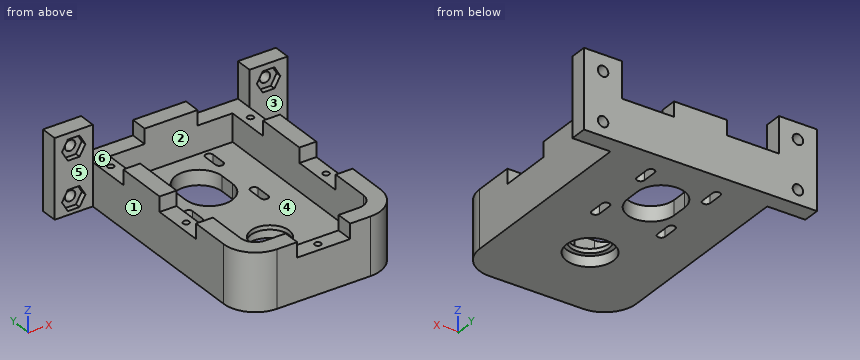
```python
from build123d import *

# Parameters (mm, degrees)
CROQUIS2_R                = 9
SALIENTE_EXTRUIR1_DEPTH   = 7
CROQUIS2_5_W              = 18
CROQUIS2_5_H              = 8
SALIENTE_EXTRUIR2_DEPTH   = 37
SALIENTE_EXTRUIR2_2_DEPTH = 37
CROQUIS2_7_W              = 25
CROQUIS2_7_H              = 8
CROQUIS2_7_W_2            = 8
CROQUIS2_7_H_2            = 25
CROQUIS2_7_H_3            = 19
CROQUIS2_7_W_3            = 9.5
SALIENTE_EXTRUIR3_DEPTH   = 27
CROQUIS2_8_W              = 8
CROQUIS2_8_H              = 25
CROQUIS2_8_W_2            = 25
CROQUIS2_8_H_2            = 8
SALIENTE_EXTRUIR4_DEPTH   = 20
CROQUIS3_R                = 11.1
CORTAR_EXTRUIR1_DEPTH     = 5
CROQUIS9_R                = 2.475
CORTAR_EXTRUIR2_DEPTH     = 2.5
CROQUIS10_R               = 2.475
CORTAR_EXTRUIR3_DEPTH     = 8
CROQUIS11_R               = 1.475
CORTAR_EXTRUIR4_DEPTH     = 7


with BuildPart() as part:
    # Croquis2 → Saliente-Extruir1 (new body)
    with BuildSketch(Plane.XY):
        with BuildLine():
            Line((-5.786620614, -56.183989891), (3.713379386, -56.183989891))
            ThreePointArc((3.713379386, -56.183989891), (8.663126854, -54.133737359), (10.713379386, -49.183989891))
            Line((10.713379386, -49.183989891), (10.713379386, -30.183989891))
            Line((10.713379386, -30.183989891), (10.713379386, -5.183989891))
            Line((10.713379386, -5.183989891), (10.713379386, 19.816010109))
            Line((10.713379386, 19.816010109), (10.713379386, 40.816010109))
            Line((10.713379386, 40.816010109), (-5.786620614, 40.816010109))
            Line((-5.786620614, 40.816010109), (-30.786620614, 40.816010109))
            Line((-30.786620614, 40.816010109), (-47.286620614, 40.816010109))
            Line((-47.286620614, 40.816010109), (-47.286620614, 19.816010109))
            Line((-47.286620614, 19.816010109), (-47.286620614, -5.183989891))
            Line((-47.286620614, -5.183989891), (-47.286620614, -30.183989891))
            Line((-47.286620614, -30.183989891), (-47.286620614, -49.183989891))
            ThreePointArc((-47.286620614, -49.183989891), (-45.236368082, -54.133737359), (-40.286620614, -56.183989891))
            Line((-40.286620614, -56.183989891), (-30.786620614, -56.183989891))
            Line((-30.786620614, -56.183989891), (-5.786620614, -56.183989891))
        make_face()
        with Locations((-18.286620614, -27.183989891)):
            Circle(CROQUIS2_R, mode=Mode.SUBTRACT)
        with BuildLine():
            ThreePointArc((-31.986620614, 6.205288522), (-33.786620614, 8.005288522), (-35.586620614, 6.205288522))
            Line((-35.586620614, 6.205288522), (-35.586620614, -0.794711478))
            ThreePointArc((-35.586620614, -0.794711478), (-33.786620614, -2.594711478), (-31.986620614, -0.794711478))
            Line((-31.986620614, -0.794711478), (-31.986620614, 6.205288522))
        make_face(mode=Mode.SUBTRACT)
        with BuildLine():
            ThreePointArc((-4.586620614, 30.205288522), (-2.786620614, 28.405288522), (-0.986620614, 30.205288522))
            Line((-0.986620614, 30.205288522), (-0.986620614, 37.205288522))
            ThreePointArc((-0.986620614, 37.205288522), (-2.786620614, 39.005288522), (-4.586620614, 37.205288522))
            Line((-4.586620614, 37.205288522), (-4.586620614, 30.205288522))
        make_face(mode=Mode.SUBTRACT)
        with BuildLine():
            ThreePointArc((-29.286620614, 14.705288522), (-18.286620614, 3.705288522), (-7.286620614, 14.705288522))
            Line((-7.286620614, 14.705288522), (-7.286620614, 21.705288522))
            ThreePointArc((-7.286620614, 21.705288522), (-18.286620614, 32.705288522), (-29.286620614, 21.705288522))
            Line((-29.286620614, 21.705288522), (-29.286620614, 14.705288522))
        make_face(mode=Mode.SUBTRACT)
        with BuildLine():
            Line((-0.986620614, 6.205288522), (-0.986620614, -0.794711478))
            ThreePointArc((-0.986620614, -0.794711478), (-2.786620614, -2.594711478), (-4.586620614, -0.794711478))
            Line((-4.586620614, -0.794711478), (-4.586620614, 6.205288522))
            ThreePointArc((-4.586620614, 6.205288522), (-2.786620614, 8.005288522), (-0.986620614, 6.205288522))
        make_face(mode=Mode.SUBTRACT)
        with BuildLine():
            Line((-35.586620614, 30.205288522), (-35.586620614, 37.205288522))
            ThreePointArc((-35.586620614, 37.205288522), (-33.786620614, 39.005288522), (-31.986620614, 37.205288522))
            Line((-31.986620614, 37.205288522), (-31.986620614, 30.205288522))
            ThreePointArc((-31.986620614, 30.205288522), (-33.786620614, 28.405288522), (-35.586620614, 30.205288522))
        make_face(mode=Mode.SUBTRACT)
    extrude(amount=SALIENTE_EXTRUIR1_DEPTH)

    # Croquis2_7 → Saliente-Extruir3 (add)
    with BuildSketch(Plane.XY):
        with Locations((-18.286620614, 44.816010109)):
            Rectangle(CROQUIS2_7_W, CROQUIS2_7_H)
        with Locations((-51.286620614, 7.316010109)):
            Rectangle(CROQUIS2_7_W_2, CROQUIS2_7_H_2)
        with Locations((-51.286620614, -39.683989891)):
            Rectangle(CROQUIS2_7_W_2, CROQUIS2_7_H_3)
        with BuildLine():
            ThreePointArc((-47.286620614, -49.183989891), (-45.236368082, -54.133737359), (-40.286620614, -56.183989891))
            Line((-40.286620614, -56.183989891), (-40.286620614, -64.183989891))
            ThreePointArc((-40.286620614, -64.183989891), (-50.893222332, -59.790591609), (-55.286620614, -49.183989891))
            Line((-55.286620614, -49.183989891), (-47.286620614, -49.183989891))
        make_face()
        with Locations((-35.536620614, -60.183989891)):
            Rectangle(CROQUIS2_7_W_3, CROQUIS2_7_H)
        with Locations((-1.036620614, -60.183989891)):
            Rectangle(CROQUIS2_7_W_3, CROQUIS2_7_H)
        with BuildLine():
            ThreePointArc((3.713379386, -56.183989891), (8.663126854, -54.133737359), (10.713379386, -49.183989891))
            Line((10.713379386, -49.183989891), (18.713379386, -49.183989891))
            ThreePointArc((18.713379386, -49.183989891), (14.319981104, -59.790591609), (3.713379386, -64.183989891))
            Line((3.713379386, -64.183989891), (3.713379386, -56.183989891))
        make_face()
        with Locations((14.713379386, -39.683989891)):
            Rectangle(CROQUIS2_7_W_2, CROQUIS2_7_H_3)
        with Locations((14.713379386, 7.316010109)):
            Rectangle(CROQUIS2_7_W_2, CROQUIS2_7_H_2)
    extrude(amount=SALIENTE_EXTRUIR3_DEPTH)



with BuildPart() as body_2:
    # Croquis2_5 → Saliente-Extruir2 (new body)
    with BuildSketch(Plane.XY):
        with Locations((27.713379386, 44.816010109)):
            Rectangle(CROQUIS2_5_W, CROQUIS2_5_H)
    extrude(amount=SALIENTE_EXTRUIR2_DEPTH)


with BuildPart() as body_3:
    # Croquis2_5 → Saliente-Extruir2 2 (new body)
    with BuildSketch(Plane.XY):
        with Locations((-64.286620614, 44.816010109)):
            Rectangle(CROQUIS2_5_W, CROQUIS2_5_H)
    extrude(amount=SALIENTE_EXTRUIR2_2_DEPTH)


with BuildPart() as part_1:
    add(part.part)

    add(body_2.part)  # Saliente-Extruir4 merges body 2

    add(body_3.part)  # Saliente-Extruir4 merges body 3
    # Croquis2_8 → Saliente-Extruir4 (add)
    with BuildSketch(Plane.XY):
        Polygon((-47.286620614, 19.816010109), (-47.286620614, 40.816010109), (-30.786620614, 40.816010109), (-30.786620614, 48.816010109), (-55.286620614, 48.816010109), (-55.286620614, 19.816010109), align=None)
        with Locations((-51.286620614, -17.683989891)):
            Rectangle(CROQUIS2_8_W, CROQUIS2_8_H)
        with Locations((-18.286620614, -60.183989891)):
            Rectangle(CROQUIS2_8_W_2, CROQUIS2_8_H_2)
        with Locations((14.713379386, -17.683989891)):
            Rectangle(CROQUIS2_8_W, CROQUIS2_8_H)
        Polygon((10.713379386, 40.816010109), (-5.786620614, 40.816010109), (-5.786620614, 48.816010109), (18.713379386, 48.816010109), (18.713379386, 19.816010109), (10.713379386, 19.816010109), align=None)
    extrude(amount=SALIENTE_EXTRUIR4_DEPTH)

    # Croquis3 → Cortar-Extruir1 (cut)
    with BuildSketch(Plane(origin=(0, 0, 0), x_dir=(-1, 0, 0), z_dir=(0, 0, -1))):
        with Locations((18.286620614, -27.183989891)):
            Circle(CROQUIS3_R)
    extrude(amount=-CORTAR_EXTRUIR1_DEPTH, mode=Mode.SUBTRACT)

    # Croquis9 → Cortar-Extruir2 (cut)
    # profile 1 of 4: a face of its own
    with BuildSketch(Plane.XZ.offset(-40.816010109)):
        Polygon((-69.826620614, 29.4), (-67.056620614, 24.602219263), (-61.516620614, 24.602219263), (-58.746620614, 29.4), (-61.516620614, 34.197780737), (-67.056620614, 34.197780737), align=None)
        with Locations(Location((-64.286620614, 29.4, 0), (0, 0, 270))):
            Circle(CROQUIS9_R, mode=Mode.SUBTRACT)
    # profile 2 of 4: a face of its own
    with BuildSketch(Plane.XZ.offset(-40.816010109)):
        Polygon((33.253379386, 6.6), (30.483379386, 11.397780737), (24.943379386, 11.397780737), (22.173379386, 6.6), (24.943379386, 1.802219263), (30.483379386, 1.802219263), align=None)
        with Locations(Location((27.713379386, 6.6, 0), (0, 0, 270))):
            Circle(CROQUIS9_R, mode=Mode.SUBTRACT)
    # profile 3 of 4: a face of its own
    with BuildSketch(Plane.XZ.offset(-40.816010109)):
        Polygon((30.483379386, 34.197780737), (33.253379386, 29.4), (30.483379386, 24.602219263), (24.943379386, 24.602219263), (22.173379386, 29.4), (24.943379386, 34.197780737), align=None)
        with Locations(Location((27.713379386, 29.4, 0), (0, 0, 90))):
            Circle(CROQUIS9_R, mode=Mode.SUBTRACT)
    # profile 4 of 4: a face of its own
    with BuildSketch(Plane.XZ.offset(-40.816010109)):
        Polygon((-67.056620614, 1.802219263), (-69.826620614, 6.6), (-67.056620614, 11.397780737), (-61.516620614, 11.397780737), (-58.746620614, 6.6), (-61.516620614, 1.802219263), align=None)
        with Locations(Location((-64.286620614, 6.6, 0), (0, 0, 90))):
            Circle(CROQUIS9_R, mode=Mode.SUBTRACT)
    extrude(amount=-CORTAR_EXTRUIR2_DEPTH, mode=Mode.SUBTRACT)

    # Croquis10 → Cortar-Extruir3 (cut)
    with BuildSketch(Plane.XZ.offset(-40.816010109)):
        with Locations(Location((-64.286620614, 29.4, 0), (0, 0, 270))):
            Circle(CROQUIS10_R)
        with Locations(Location((-64.286620614, 6.6, 0), (0, 0, 270))):
            Circle(CROQUIS10_R)
        with Locations(Location((27.713379386, 29.4, 0), (0, 0, 270))):
            Circle(CROQUIS10_R)
        with Locations(Location((27.713379386, 6.6, 0), (0, 0, 270))):
            Circle(CROQUIS10_R)
    extrude(amount=-CORTAR_EXTRUIR3_DEPTH, mode=Mode.SUBTRACT)

    # Croquis11 → Cortar-Extruir4 (cut)
    with BuildSketch(Plane.XY.offset(20)):
        with Locations((-51.286620614, 34.316010109)):
            Circle(CROQUIS11_R)
        with Locations((-51.286620614, -17.683989891)):
            Circle(CROQUIS11_R)
        with Locations((-18.286620614, -60.183989891)):
            Circle(CROQUIS11_R)
        with Locations(Location((14.713379386, -17.683989891, 0), (0, 0, 180))):
            Circle(CROQUIS11_R)
        with Locations(Location((14.713379386, 34.316010109, 0), (0, 0, 180))):
            Circle(CROQUIS11_R)
    extrude(amount=-CORTAR_EXTRUIR4_DEPTH, mode=Mode.SUBTRACT)


solid = part_1.part
```
The listing builds one solid part. Answer for the finished solid, in the listing's coordinates (mm). Face numbers are marked on the shaded views. A direction names the side the tool comes from. Give positions to 0.01 mm unless a question says otherwise; leave off trailing zeros. Loops run counter-clockwise (first coordinate to the right, second up) from the corner with the lowest first, then second, coordinate; pieces in that order, holes last. Notation, with made-up numbers: M 63,56 L 86,56 A30 ccw 86,82 Z; hole C 28,10 d11. An arc over 180 degrees is marked long. One line per item, written item: value.
1. For the marked faces 4, 5 and 6, determine the directions among +Z, -Z, +X, -X, +Y, -Y from which every point of the face is accessible in a straight line to the end or side of a thin tool.
Found:
face 4: +Z
face 5: +Z, -Z, -X, -Y
face 6: +Z, +Y
2. Section A-A on x = -22 is taken. Determine the outline of the cut face in (y, z), plus the area to 3 significant figures.
Found:
outline: M -64.18,0 L -37.64,0 L -37.64,5 L -35.38,5 L -35.38,7 L -56.18,7 L -56.18,20 L -64.18,20 Z; M -18.99,5 L -16.72,5 L -16.72,0 L 4.35,0 L 4.35,7 L -18.99,7 Z; M 32.06,0 L 48.82,0 L 48.82,27 L 40.82,27 L 40.82,7 L 32.06,7 Z
area: 724 mm^2
3. For a pull along Y with two mould halves and no side action, classify the marked faces 1, 2 and 3 as pulls with the +Y half, pulls with the -Y half, needs draft (parallel to the pull), parting line crosses it, or undercut.
Found:
face 1: needs draft
face 2: undercut
face 3: pulls with the -Y half
4. Find the intervals of material crossed by probe 1 along X at (y, z) = (47, 29.4); probe 2 along Y at (x, z) = (-10, 12); probe 3 along X at (y, z) = (43.5, 5), in increasing order.
Found:
probe 1: -73.29 to -66.76, -61.81 to -55.29, 18.71 to 25.24, 30.19 to 36.71
probe 2: -64.18 to -56.18, 40.82 to 48.82
probe 3: -73.29 to -66.17, -62.4 to 25.83, 29.6 to 36.71
5. Each of these flat-tipped pins is pushed along its axis until it touches: P1, Ø1, axis at y = -46, z = 14.5, coming from the -X side; P2, Ø10, axis at y = 29.5, z = 21, coming from the +X side; P3, Ø7.5, axis at x = -52, z = 25, coming from the -Y side. Where does it stop, or does it pass through?
Found:
P1: x = -55.29
P2: x = 18.71
P3: y = -61.9
6. Section C-C on z = 14.5 is taken. Determine the outline of the cut face in (x, y) (3 decimals).
Found:
outline: M -73.287,40.816 L -55.287,40.816 L -55.287,-49.184 A15 ccw -40.287,-64.184 L 3.713,-64.184 A15 ccw 18.713,-49.184 L 18.713,40.816 L 36.713,40.816 L 36.713,48.816 L -73.287,48.816 Z; hole C -51.287,-17.684 d2.95; hole C -51.287,34.316 d2.95; hole M -47.287,-49.184 A7 ccw -40.287,-56.184 L 3.713,-56.184 A7 ccw 10.713,-49.184 L 10.713,40.816 L -47.287,40.816 Z; hole C -18.287,-60.184 d2.95; hole C 14.713,-17.684 d2.95; hole C 14.713,34.316 d2.95
7. Section B-B on z = 23 is taken. State how many separate pieces and enclosed holes the cut face has, plus the area to 3 significant figures.
Found:
separate pieces: 7
enclosed holes: 0
area: 1,620 mm^2
